```python
from build123d import *

# Parameters (mm, degrees)
BOSS_EXTRUDE1_DEPTH                  = 12.337299938
SKETCH2_R                            = 6.35
BOSS_EXTRUDE2_DEPTH                  = 7.9375
F_10_32_TAPPED_HOLE1_D               = 4.0386
F_10_32_TAPPED_HOLE1_DEPTH           = 15.07744
F_10_32_TAPPED_HOLE1_TIP             = 1.213317848
F_10_32_TAPPED_HOLE1_ON_FACE_2_D     = 4.0386
F_10_32_TAPPED_HOLE1_ON_FACE_2_DEPTH = 15.07744
F_10_32_TAPPED_HOLE1_ON_FACE_2_TIP   = 1.213317848


with BuildPart() as part:
    # Sketch1 → Boss-Extrude1 (new, symmetric)
    with BuildSketch(Plane.XY):
        with BuildLine():
            ThreePointArc((6.35, 2.590301913), (5.939202219, 3.429), (5.41826726, 4.204110358))
            Line((5.41826726, 4.204110358), (0.93173274, 6.79441227))
            ThreePointArc((0.93173274, 6.79441227), (0, 6.858), (-0.93173274, 6.79441227))
            Line((-0.93173274, 6.79441227), (-5.41826726, 4.204110358))
            ThreePointArc((-5.41826726, 4.204110358), (-5.939202219, 3.429), (-6.35, 2.590301913))
            Line((-6.35, 2.590301913), (-6.35, -2.590301913))
            ThreePointArc((-6.35, -2.590301913), (-5.939202219, -3.429), (-5.41826726, -4.204110358))
            Line((-5.41826726, -4.204110358), (-0.93173274, -6.79441227))
            ThreePointArc((-0.93173274, -6.79441227), (0, -6.858), (0.93173274, -6.79441227))
            Line((0.93173274, -6.79441227), (5.41826726, -4.204110358))
            ThreePointArc((5.41826726, -4.204110358), (5.939202219, -3.429), (6.35, -2.590301913))
            Line((6.35, -2.590301913), (6.35, 2.590301913))
        make_face()
    extrude(amount=BOSS_EXTRUDE1_DEPTH, both=True)

    # Sketch2 → Boss-Extrude2 (add)
    with BuildSketch(Plane.XY.offset(12.337299938)):
        Circle(SKETCH2_R)
    boss_extrude2 = extrude(amount=BOSS_EXTRUDE2_DEPTH)

    # Mirror1: Boss-Extrude2 across plane
    add(boss_extrude2.mirror(Plane.XY))

    # #10-32 Tapped Hole1
    with Locations(Plane.XY.offset(20.274799938)):
        with Locations((0, 0)):
            Hole(F_10_32_TAPPED_HOLE1_D / 2, depth=F_10_32_TAPPED_HOLE1_DEPTH)
            with Locations((0, 0, -(F_10_32_TAPPED_HOLE1_DEPTH + F_10_32_TAPPED_HOLE1_TIP / 2))):  # 118° drill point
                Cone(0, F_10_32_TAPPED_HOLE1_D / 2, F_10_32_TAPPED_HOLE1_TIP, mode=Mode.SUBTRACT)

    # #10-32 Tapped Hole1 on face 2
    with Locations(Plane(origin=(0, 0, -20.274799938), x_dir=(-1, 0, 0), z_dir=(0, 0, -1))):
        with Locations((0, 0)):
            Hole(F_10_32_TAPPED_HOLE1_ON_FACE_2_D / 2, depth=F_10_32_TAPPED_HOLE1_ON_FACE_2_DEPTH)
            with Locations((0, 0, -(F_10_32_TAPPED_HOLE1_ON_FACE_2_DEPTH + F_10_32_TAPPED_HOLE1_ON_FACE_2_TIP / 2))):  # 118° drill point
                Cone(0, F_10_32_TAPPED_HOLE1_ON_FACE_2_D / 2, F_10_32_TAPPED_HOLE1_ON_FACE_2_TIP, mode=Mode.SUBTRACT)


solid = part.part
```
Read the model definition and answer for the solid it produces. Units are mm, in the model's axes. A direction names the side the tool comes from. Give positions to 0.01 mm unless a question says otherwise; leave off trailing zeros. Write each loop counter-clockwise with the first axis right and the second up, starting at its lowest first coordinate (ties: lowest second). Pieces come first, ordered by that corner, then holes. Notation, with made-up numbers: (-17, 61.25) - (36, 61.25) arc R8 cw to (36, 66.25) - close; hole circle Ø1 at (58.5, 15.25). An arc over 180 degrees is marked (long way). Write item = value, one per line. Start each with the question number.
Item 1: Find the intervals of material crossed by probe 1 along X at (y, z) = (0, 11), in increasing order. Write a range as [from, to].
Item 2: Find section B-B (z = 1). Give the vertices of the cut face in (x, y), then the cut area to 3 significant figures.
Item 3: Each of these flat-tipped pins is pushed along its axis until it touches: P1, Ø4, axis at x = 2.5, z = 16, coming from the -Y side; P2, Ø4, axis at x = 4.5, z = 7.5, coming from the +Y side; P3, Ø3, axis at x = 0, y = 0, coming from the +Z side. Where does it stop, or does it pass through?
Item 4: Find section A-A (z = 8). Give the vertices of the cut face in (x, y).
Item 5: The mould has two halves that part along X. Classify faces 1 (the flat face through (6.35, 0, 0)), 2 (the conical face through (-0.076, -0.342, 4.195)), 3 (the flat face through (-5.7, 3.2, 12.337)), 4 (the cylindrical face through (0.013, 6.858, 0.173)): +X half, -X half, draft (parallel to the pull), parting line (faces both ways), or undercut.
Item 6: Find section C-C (x = -4). Give the vertices of the cut face in (y, z).
Item 7: A tool of negligible diameter and unlimited length cuts with its end or side. For faces 5 (the flat face through (5.7, 3.2, 12.337)), 6 (the flat face through (5.7, 3.2, -12.337)), 7 (the flat face through (0, 6.5, -12.337)), 8 (the flat face through (-5.6, -3.3, 12.337)), from which of +Z, -Z, +X, -X, +Y, -Y can it reach the whole face along a straight path? Write none if from no direction.
Response:
q1.probe_1 = [-6.35, -2.02], [2.02, 6.35]
q2.outline = (-6.35, -2.59) arc R6.86 ccw to (-5.42, -4.2) - (-0.93, -6.79) arc R6.86 ccw to (0.93, -6.79) - (5.42, -4.2) arc R6.86 ccw to (6.35, -2.59) - (6.35, 2.59) arc R6.86 ccw to (5.42, 4.2) - (0.93, 6.79) arc R6.86 ccw to (-0.93, 6.79) - (-5.42, 4.2) arc R6.86 ccw to (-6.35, 2.59) - close
q2.area = 137 mm²
q3.P1 = -6.33
q3.P2 = 5.89
q3.P3 = 4.89
q4.outline = (-6.35, -2.59) arc R6.86 ccw to (-5.42, -4.2) - (-0.93, -6.79) arc R6.86 ccw to (0.93, -6.79) - (5.42, -4.2) arc R6.86 ccw to (6.35, -2.59) - (6.35, 2.59) arc R6.86 ccw to (5.42, 4.2) - (0.93, 6.79) arc R6.86 ccw to (-0.93, 6.79) - (-5.42, 4.2) arc R6.86 ccw to (-6.35, 2.59) - close; hole circle Ø4.04 at (0, 0)
q5.face_1 = +X half
q5.face_2 = undercut
q5.face_3 = draft
q5.face_4 = parting line
q6.outline = (-5.02, -12.34) - (-4.93, -12.34) - (-4.93, -20.27) - (4.93, -20.27) - (4.93, -12.34) - (5.02, -12.34) - (5.02, 12.34) - (4.93, 12.34) - (4.93, 20.27) - (-4.93, 20.27) - (-4.93, 12.34) - (-5.02, 12.34) - close
q7.face_5 = +Z, +X, +Y
q7.face_6 = -Z, +X, +Y
q7.face_7 = -Z, +Y
q7.face_8 = +Z, -X, -Y
